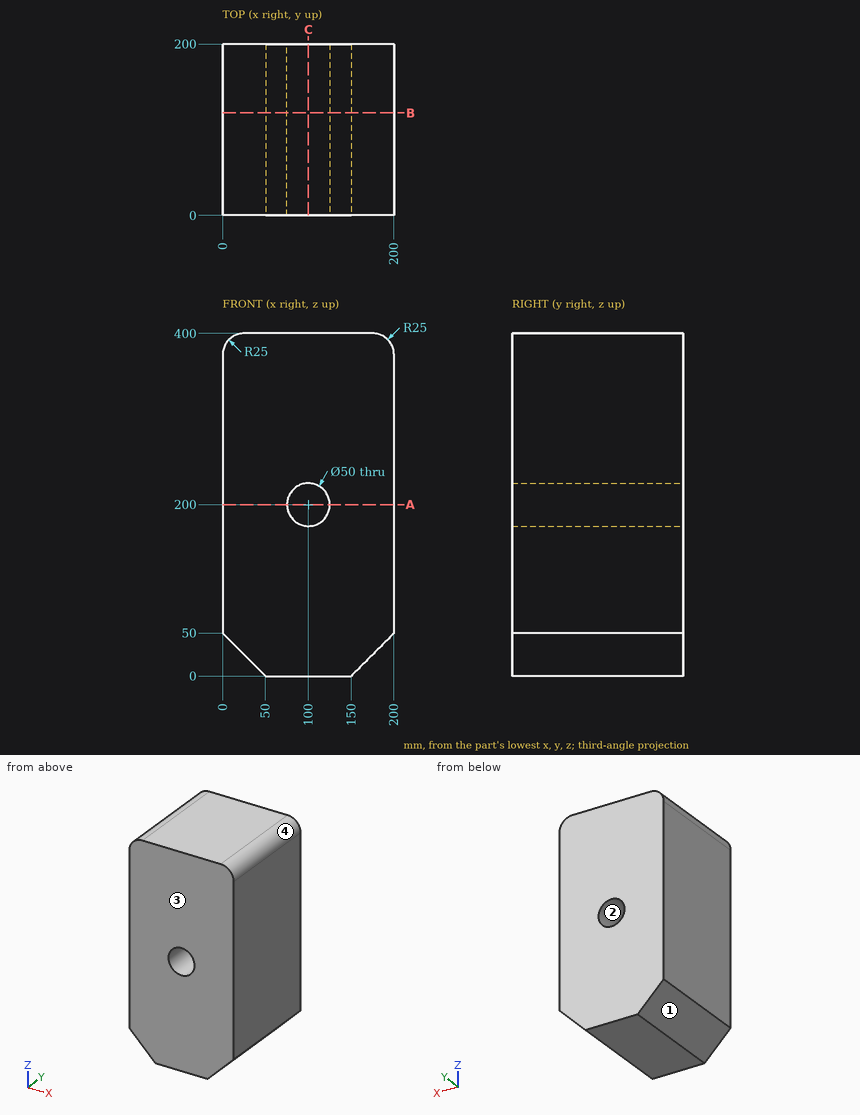
Job drawing, mm, ordinate dimensions from the low corner. One solid piece. Give positions to 0.01 mm unless a question says otherwise; leave off trailing zeros. Loops run counter-clockwise (first coordinate to the right, second up) from the corner with the lowest first, then second, coordinate; pieces in that order, holes last. Notation, with made-up numbers: M -19,55.5 L -1,55.5 A15 cw -1,68.5 Z; hole C -17,-8 d4. An arc over 180 degrees is marked long. Put each result on its own line as item: value. Start each with the question number.
1) Pull direction X, two halves, no side cores. Call the marked faces 1, 2, 3 and 4: +X half, -X half, draft (parallel to the pull), parting line (faces both ways), or undercut.
2) Saw through at B-B (y = 119.5). List the corners of the cut face in (x, z), then the cut area to 3 significant figures.
3) Saw through at A-A (z = 200). List the corners of the cut face in (x, y).
4) Saw through at C-C (x = 100). List the corners of the cut face in (y, z), then the cut area to 3 significant figures.
5) Probe probe 1 along Z at (x, y) = (100, 48); probe 2 along X at (y, z) = (153, 182); probe 3 along X at (y, z) = (56, 39). List the from-to ranges inside material, lowest first.
Numbers:
1. face 1: -X half
1. face 2: undercut
1. face 3: draft
1. face 4: +X half
2. outline: M 0,50 L 50,0 L 150,0 L 200,50 L 200,375 A25 ccw 175,400 L 25,400 A25 ccw 0,375 Z; hole C 100,200 d50
2. area: 75,300 mm^2
3. outline: M 0,0 L 75,0 L 75,200 L 0,200 Z; M 125,0 L 200,0 L 200,200 L 125,200 Z
4. outline: M 0,0 L 200,0 L 200,175 L 0,175 Z; M 0,225 L 200,225 L 200,400 L 0,400 Z
4. area: 70,000 mm^2
5. probe 1: 0 to 175, 225 to 400
5. probe 2: 0 to 82.65, 117.35 to 200
5. probe 3: 11 to 189
